Verification items for the finished model (mm, model axes). A direction names the side the tool comes from. Give positions to 0.01 mm unless a question says otherwise; leave off trailing zeros. Loops run counter-clockwise (first coordinate to the right, second up) from the corner with the lowest first, then second, coordinate; pieces in that order, holes last. Notation, with made-up numbers: M -21,-27 L -11,-27 A11 ccw -11,-13 Z; hole C 69.5,22 d1. An arc over 180 degrees is marked long. Answer in a Markdown table with one row per item.
```python
from build123d import *

# Parameters (mm, degrees)
F1_DEPTH      = 7.62
F1_DEPTH_BACK = 38.1
F2_DEPTH      = 15.24
F3_W          = 30.48
F3_H          = 15.24
F4_DEPTH      = 152.4
F5_R          = 1.27
F5_R_2        = 1.2522055882
F6_DEPTH      = 25.4


# Not quite as in the source:
# - a feature names something its author has since deleted; it is built from what else it names


with BuildPart() as f1:
    # F0 (on Right) → F1 (new body, two sides)
    with BuildSketch(Plane.YZ) as f1_sk:
        Polygon((-19.9023338153, 49.1049804437), (-37.6823338153, 49.1049804437), (-37.6823338153, -16.8750494665), (-19.9023338153, -20.654305133), align=None)
        Polygon((-37.6823338153, 49.1049804437), (-45.3023338153, 49.1049804437), (-45.3023338153, -15.2553684666), (-37.6823338153, -16.8750494665), align=None)
    extrude(amount=F1_DEPTH)
    extrude(f1_sk.sketch, amount=-F1_DEPTH_BACK)

    # F0 (on Right) → F2 (join)
    with BuildSketch(Plane.YZ):
        Polygon((-37.6823338153, 49.1049804437), (-45.3023338153, 49.1049804437), (-45.3023338153, -15.2553684666), (-37.6823338153, -16.8750494665), align=None)
    extrude(amount=-F2_DEPTH)

    # F3 (on face) → F4 (cut)
    with BuildSketch(Plane.XY.offset(49.1049804437)):
        with Locations((-15.24, -27.5223338153)):
            Rectangle(F3_W, F3_H)
    extrude(amount=-F4_DEPTH, mode=Mode.SUBTRACT)

    # F5 (on face) → F6 (join)
    with BuildSketch(Plane(origin=(0, -5.0607549484, -23.8089801067), x_dir=(1, 0, 0), z_dir=(0, -0.2079116908, -0.9781476007))):
        with Locations((-28.575, 32.6586192333)):
            Circle(F5_R)
        with Locations((-1.905, 32.6586192333)):
            Circle(F5_R_2)
    extrude(amount=F6_DEPTH)


solid = f1.part
```
Item 1: Release check for a two-part mould opening along Z. For faces 3 (the cylindrical face through (-27.402, -39.133, -29.369)), 4 (the cylindrical face through (-2.176, -38.414, -29.522)), 5 (the flat face through (0, -28, 15)), 6 (the flat face through (-28.59, -42.3, -41.86)) record: released by +Z, released by -Z, zero draft, split by the parting line, or undercut.
Reported:
| item | result |
|---|---|
| face 3 | undercut |
| face 4 | undercut |
| face 5 | zero draft |
| face 6 | released by -Z |
Item 2: Scan lines: L1, parallel to X at y = -31, z = 28; L2, parallel to X at y = -39, z = -26; L3, parallel to Y at x = -11, z = -2.5. Record each from-to range of solid material in increasing order. Write a range as [from, to].
Reported:
| item | result |
|---|---|
| L1 | x = [-38.1, -30.48], [0, 7.62] |
| L2 | x = [-29.84, -27.31], [-3.15, -0.66] |
| L3 | y = [-45.3, -35.14] |
Item 3: Tool access check on faces 1 (the flat face through (-15, -35.142, 16)), 2 (the flat face through (-38.1, -33, 15)). Record the directions out of +Z, -Z, +X, -X, +Y, -Y that give a thin tool (end or side, any length) a straight path to the whole face; none if there is none.
Reported:
| item | result |
|---|---|
| face 1 | +Z, -Z, +Y |
| face 2 | +Z, -Z, -X, +Y, -Y |
Item 4: Go/stop test with flat-tipped pins: pin 1 (6 mm diameter, centred on x = -1.5, y = -33.5, fed in from +Z) (3 decimals); pin 2 (3 mm diameter, centred on x = -19, y = -41.5, fed in from -Z); pin 3 (15 mm diameter, centred on x = -18.5, z = 29.5, fed in from +Y). Record where each tip stops, or that it passes through.
Reported:
| item | result |
|---|---|
| pin 1 | stops at z = 49.105 |
| pin 2 | stops at z = -16.38 |
| pin 3 | stops at y = -35.14 |
Item 5: Sectioned sample at A-A (y = -30.75). Record the cut outline in (x, z).
Reported:
| item | result |
|---|---|
| outline | M -38.1,-18.35 L -30.48,-18.35 L -30.48,49.1 L -38.1,49.1 Z; M 0,-18.35 L 7.62,-18.35 L 7.62,49.1 L 0,49.1 Z |
Item 6: Sectioned sample at D-D (x = 5). Record the cut outline in (y, z), and give its area (3 significant figures).
Reported:
| item | result |
|---|---|
| outline | M -45.3,-15.26 L -19.9,-20.65 L -19.9,49.1 L -45.3,49.1 Z |
| area | 1,700 mm^2 |
Item 7: Sectioned sample at B-B (z = -1.5). Record the cut outline in (x, y).
Reported:
| item | result |
|---|---|
| outline | M -38.1,-45.3 L 7.62,-45.3 L 7.62,-19.9 L 0,-19.9 L 0,-35.14 L -30.48,-35.14 L -30.48,-19.9 L -38.1,-19.9 Z |
Item 8: Sectioned sample at C-C (x = -9.5). Record the cut outline in (y, z), and give its area (3 significant figures).
Reported:
| item | result |
|---|---|
| outline | M -45.3,-15.26 L -35.14,-17.41 L -35.14,49.1 L -45.3,49.1 Z |
| area | 665 mm^2 |
